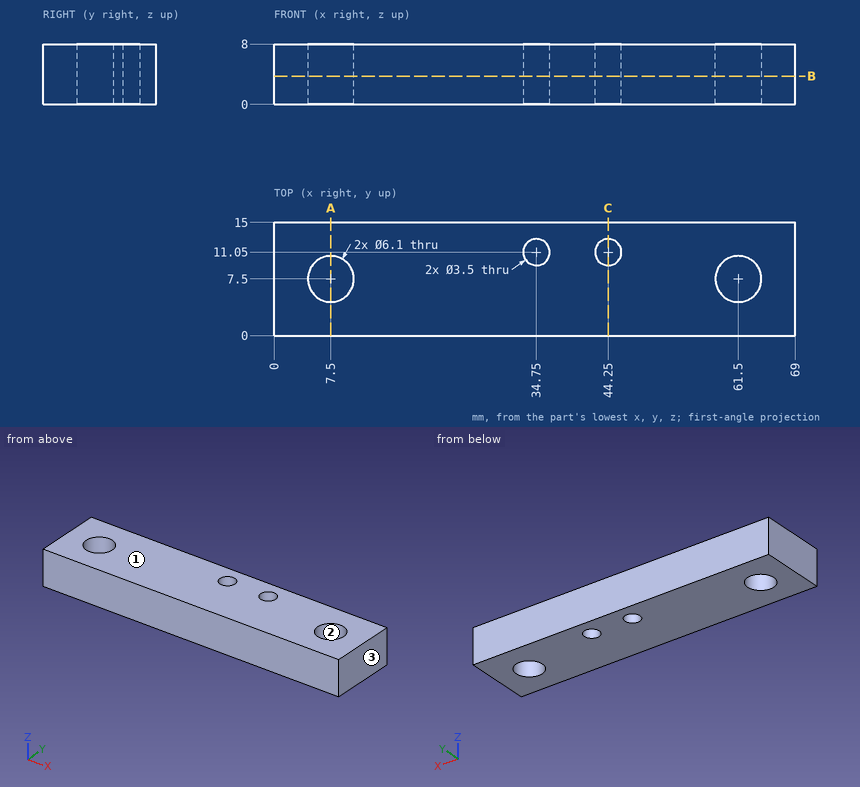
Here's the drawing with two shaded views (mm, measured from the low corner). I have some questions. Give positions to 0.01 mm unless a question says otherwise; leave off trailing zeros. Loops run counter-clockwise (first coordinate to the right, second up) from the corner with the lowest first, then second, coordinate; pieces in that order, holes last. Notation, with made-up numbers: M -22.75,-39 L 32.25,-39 A11 cw 32.25,-22 Z; hole C -26.5,-26.5 d5. An arc over 180 degrees is marked long. Use one line per item in the form item = value. Start each with the question number.
Q1. I need wall thicknesses on line 1 along Y through (x, z) = (7.5, 5); line 2 along X through (y, z) = (7.75, 1.75); line 3 along Y through (x, z) = (44.25, 6). Which ranges of each line are inside material? Lowest first, please.
Q2. Thinking about a two-plate mould opening in X: for the marked faces 1, 2 and 3, which applies, +X half, -X half, draft (parallel to the pull), parting line (faces both ways), or undercut?
Q3. If we section it at C-C (x = 44.25): Write out the boundary of the cut face in (y, z), then the cut area to 3 significant figures.
Q4. If we section it at A-A (x = 7.5): Write out the boundary of the cut face in (y, z).
Q5. If we section it at B-B (z = 3.75): Write out the boundary of the cut face in (x, y), then the cut area to 3 significant figures.
Taken from the geometry:
q1.line_1 = 0 to 4.45, 10.55 to 15
q1.line_2 = 0 to 4.46, 10.54 to 58.46, 64.54 to 69
q1.line_3 = 0 to 9.3, 12.8 to 15
q2.face_1 = draft
q2.face_2 = undercut
q2.face_3 = +X half
q3.outline = M 0,0 L 9.3,0 L 9.3,8 L 0,8 Z; M 12.8,0 L 15,0 L 15,8 L 12.8,8 Z
q3.area = 92.0 mm^2
q4.outline = M 0,0 L 4.45,0 L 4.45,8 L 0,8 Z; M 10.55,0 L 15,0 L 15,8 L 10.55,8 Z
q5.outline = M 0,0 L 69,0 L 69,15 L 0,15 Z; hole C 7.5,7.5 d6.1; hole C 34.75,11.05 d3.5; hole C 44.25,11.05 d3.5; hole C 61.5,7.5 d6.1
q5.area = 957 mm^2
